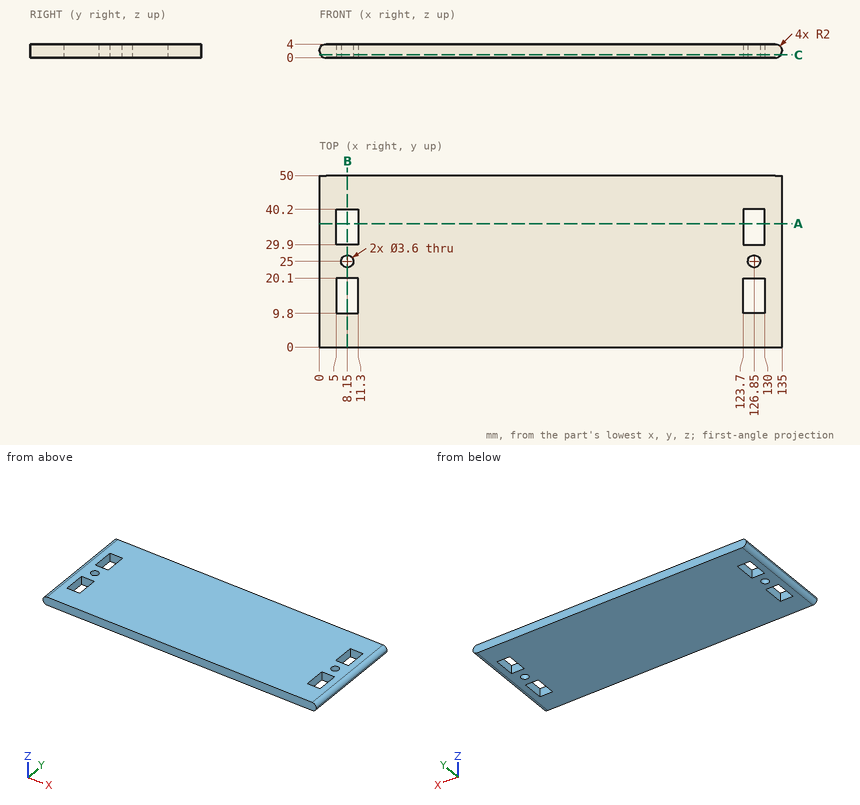
Check sheet for the drawn part. Datum: minimum x, y, z corner. Units: mm. Give positions to 0.01 mm unless a question says otherwise; leave off trailing zeros. Write each loop counter-clockwise with the first axis right and the second up, starting at its lowest first coordinate (ties: lowest second). Pieces come first, ordered by that corner, then holes. Notation, with made-up numbers: (-16, -38) -> (35, -38) arc R28 cw to (35, -4) -> close; hole circle Ø1 at (80, 84). An arc over 180 degrees is marked (long way). Use one line per item in the form item = value. Start each with the question number.
1. Thickness scan on line 1 along Y through (x, z) = (8.15, 1.35); line 2 along X through (y, z) = (17.5, 2); line 3 along X through (y, z) = (38, 0.4). Record the ranges inside material, lowest first. Write a range as from..to.
2. Go/stop test with flat-tipped pins: P1, Ø3, axis at x = 126.85, y = 25, coming from the +Z side; P2, Ø1, axis at y = 8, z = 3.5, coming from the +X side. Record where each tip stops, or that it passes through.
3. Section check B-B (x = 8.15). Record the cut outline in (y, z), and give its area (3 significant figures).
4. Section check A-A (y = 36). Count the separate pieces of the cut face and the enclosed holes in it, and give its area (3 significant figures).
5. Section check C-C (z = 0.8). Record the cut outline in (x, y).
Conclusion:
q1.line_1 = 0..9.8, 20.1..23.2, 26.8..29.9, 40.2..50
q1.line_2 = 0..5, 11.3..123.7, 130..135
q1.line_3 = 0.8..5, 11.3..123.7, 130..134.2
q2.P1 = through
q2.P2 = 134.73
q3.outline = (0, 0) -> (9.8, 0) -> (9.8, 4) -> (0, 4) -> close; (20.1, 0) -> (23.2, 0) -> (23.2, 4) -> (20.1, 4) -> close; (26.8, 0) -> (29.9, 0) -> (29.9, 4) -> (26.8, 4) -> close; (40.2, 0) -> (50, 0) -> (50, 4) -> (40.2, 4) -> close
q3.area = 103 mm²
q4.separate_pieces = 3
q4.enclosed_holes = 0
q4.area = 486 mm²
q5.outline = (0.4, 0) -> (134.6, 0) -> (134.6, 50) -> (0.4, 50) -> close; hole (5, 9.8) -> (11.3, 9.8) -> (11.3, 20.1) -> (5, 20.1) -> close; hole (5, 29.9) -> (11.3, 29.9) -> (11.3, 40.2) -> (5, 40.2) -> close; hole circle Ø3.6 at (8.15, 25); hole (123.7, 9.8) -> (130, 9.8) -> (130, 20.1) -> (123.7, 20.1) -> close; hole (123.7, 29.9) -> (130, 29.9) -> (130, 40.2) -> (123.7, 40.2) -> close; hole circle Ø3.6 at (126.85, 25)
